```python
from build123d import *

# Parameters (mm, degrees)
F0_R     = 3.175
F1_DEPTH = 3.048


with BuildPart() as f1:
    # F0 (on Front) → F1 (new body)
    with BuildSketch(Plane.XZ):
        with BuildLine():
            Line((0.6794904459, -9.5007324841), (0, -9.525))
            ThreePointArc((0, -9.525), (0.3399618281, -9.5189311877), (0.6794904459, -9.5007324841))
        make_face()
        with BuildLine():
            Line((-15.7474569047, 61.4917106696), (-9.4773410414, -0.9516468803))
            ThreePointArc((-9.4773410414, -0.9516468803), (-7.0636414665, 6.3898821767), (0, 9.525))
            Line((0, 9.525), (0, 47.625))
            ThreePointArc((0, 47.625), (-10.4912828548, 51.5857812233), (-15.7474569047, 61.4917106696))
        make_face()
        with BuildLine():
            ThreePointArc((9.525, 0), (6.9712901065, -6.4905114784), (0.6794904459, -9.5007324841))
            Line((0.6794904459, -9.5007324841), (44.45, -7.9375))
            ThreePointArc((44.45, -7.9375), (38.8373399243, -5.6126600757), (36.5125, 0))
            Line((36.5125, 0), (9.525, 0))
        make_face()
        with BuildLine():
            Line((0, 104.775), (0, 79.375))
            ThreePointArc((0, 79.375), (10.4912828548, 75.4142187767), (15.7474569047, 65.5082893304))
            Line((15.7474569047, 65.5082893304), (9.525, 114.3))
            ThreePointArc((9.525, 114.3), (6.7351920908, 107.5648079092), (0, 104.775))
        make_face()
        with BuildLine():
            ThreePointArc((9.525, 114.3), (0, 123.825), (-9.525, 114.3))
            ThreePointArc((-9.525, 114.3), (-6.7351920908, 107.5648079092), (0, 104.775))
            ThreePointArc((0, 104.775), (6.7351920908, 107.5648079092), (9.525, 114.3))
        make_face()
        with BuildLine():
            ThreePointArc((3.175, 114.3), (2.2450640303, 112.0549359697), (0, 111.125))
            ThreePointArc((0, 111.125), (-2.2450640303, 116.5450640303), (3.175, 114.3))
        make_face(mode=Mode.SUBTRACT)
        with BuildLine():
            ThreePointArc((36.5125, 0), (38.8373399243, -5.6126600757), (44.45, -7.9375))
            ThreePointArc((44.45, -7.9375), (50.0626600757, -5.6126600757), (52.3875, 0))
            ThreePointArc((52.3875, 0), (50.0626600757, 5.6126600757), (44.45, 7.9375))
            ThreePointArc((44.45, 7.9375), (38.8373399243, 5.6126600757), (36.5125, 0))
        make_face()
        with BuildLine():
            ThreePointArc((47.625, 0), (44.45, -3.175), (41.275, 0))
            ThreePointArc((41.275, 0), (44.45, 3.175), (47.625, 0))
        make_face(mode=Mode.SUBTRACT)
        with BuildLine():
            Line((0, 60.325), (0, 47.625))
            ThreePointArc((0, 47.625), (10.4912828548, 51.5857812233), (15.7474569047, 61.4917106696))
            ThreePointArc((15.7474569047, 61.4917106696), (15.8430821396, 62.4938323604), (15.875, 63.5))
            ThreePointArc((15.875, 63.5), (15.8430821396, 64.5061676396), (15.7474569047, 65.5082893304))
            ThreePointArc((15.7474569047, 65.5082893304), (10.4912828548, 75.4142187767), (0, 79.375))
            Line((0, 79.375), (0, 66.675))
            ThreePointArc((0, 66.675), (2.2450640303, 65.7450640303), (3.175, 63.5))
            ThreePointArc((3.175, 63.5), (2.2450640303, 61.2549359697), (0, 60.325))
        make_face()
        with BuildLine():
            ThreePointArc((-15.7474569047, 65.5082893304), (-15.875, 63.5), (-15.7474569047, 61.4917106696))
            ThreePointArc((-15.7474569047, 61.4917106696), (-10.4912828548, 51.5857812233), (0, 47.625))
            Line((0, 47.625), (0, 60.325))
            ThreePointArc((0, 60.325), (-3.175, 63.5), (0, 66.675))
            Line((0, 66.675), (0, 79.375))
            ThreePointArc((0, 79.375), (-10.4912828548, 75.4142187767), (-15.7474569047, 65.5082893304))
        make_face()
        with BuildLine():
            Line((-9.525, 114.3), (-15.7474569047, 65.5082893304))
            ThreePointArc((-15.7474569047, 65.5082893304), (-10.4912828548, 75.4142187767), (0, 79.375))
            Line((0, 79.375), (0, 104.775))
            ThreePointArc((0, 104.775), (-6.7351920908, 107.5648079092), (-9.525, 114.3))
        make_face()
        with Locations((-6.35, 100.0252)):
            Circle(F0_R, mode=Mode.SUBTRACT)
        with BuildLine():
            Line((0, 47.625), (0, 9.525))
            ThreePointArc((0, 9.525), (6.7351920908, 6.7351920908), (9.525, 0))
            Line((9.525, 0), (36.5125, 0))
            ThreePointArc((36.5125, 0), (38.8373399243, 5.6126600757), (44.45, 7.9375))
            Line((44.45, 7.9375), (17.7825532299, 8.8935802069))
            ThreePointArc((17.7825532299, 8.8935802069), (12.0075791655, 11.6923910174), (10.1810740488, 17.8444269776))
            Line((10.1810740488, 17.8444269776), (15.7474569047, 61.4917106696))
            ThreePointArc((15.7474569047, 61.4917106696), (10.4912828548, 51.5857812233), (0, 47.625))
        make_face()
        with BuildLine():
            ThreePointArc((0, 9.525), (-7.0636414665, 6.3898821767), (-9.4773410414, -0.9516468803))
            ThreePointArc((-9.4773410414, -0.9516468803), (-6.3898821767, -7.0636414665), (0, -9.525))
            Line((0, -9.525), (0.6794904459, -9.5007324841))
            ThreePointArc((0.6794904459, -9.5007324841), (6.9712901065, -6.4905114784), (9.525, 0))
            Line((9.525, 0), (3.175, 0))
            ThreePointArc((3.175, 0), (-2.2450640303, -2.2450640303), (0, 3.175))
            Line((0, 3.175), (0, 9.525))
        make_face()
        with BuildLine():
            ThreePointArc((9.525, 0), (6.7351920908, 6.7351920908), (0, 9.525))
            Line((0, 9.525), (0, 3.175))
            ThreePointArc((0, 3.175), (2.2450640303, 2.2450640303), (3.175, 0))
            Line((3.175, 0), (9.525, 0))
        make_face()
    extrude(amount=F1_DEPTH)


solid = f1.part
```
Geometry: final body of the model. Coordinates: model frame, mm. A direction names the side the tool comes from. Coordinates: 2 decimals unless noted, no trailing zeros. Order: outer loops, then holes, each group sorted by start corner. A loop starts at its lowest first (then second) coordinate and runs counter-clockwise, first axis right, second up. Notation, with made-up numbers: (47, 5.25) - (91, 5.25) arc R20 cw to (91, 35.25) - close; hole circle Ø8 at (74, -3.75). An arc over 180 degrees is marked (long way). Write each question's results on one line, items separated by ' | '.
(1) Set-up query: faces 5 (the face through (0.209, -1.503, 123.823)), 6 (the face through (12.925, -1.503, 39.363)). Return all of +Z, -Z, +X, -X, +Y, -Y with unobstructed straight access to the full face (end or side cutting, diameter ignored); none if empty.
Values found:
face 5: +Z, +Y, -Y | face 6: +X, +Y, -Y
(2) Line query: line 1 (Z direction, x = -2, y = -2.8); line 2 (X direction, y = -0.85, z = 114.3) (3 decimals); line 3 (Z direction, x = -0.5, y = -0.75). Output: solid intervals per line, ascending. Write a range as [from, to].
Values found:
line 1: z = [-9.31, -2.47], [2.47, 61.03], [65.97, 111.83], [116.77, 123.61] | line 2: x = [-9.525, -3.175], [3.175, 9.525] | line 3: z = [-9.51, -3.14], [3.14, 60.36], [66.64, 111.16], [117.44, 123.81]
(3) Section query B-B, the plane z = 84.5. Return the cut outline in (x, y), plus the area to 3 significant figures.
Values found:
outline: (-13.33, -3.05) - (13.33, -3.05) - (13.33, 0) - (-13.33, 0) - close | area: 81.2 mm²
(4) Section query A-A, the plane y = -2.35. Count the separate pieces of the cut face and the enclosed holes in it, plus the area to 3 significant figures.
Values found:
separate pieces: 1 | enclosed holes: 5 | area: 3,730 mm²
(5) Mould query, pull axis X, two halves, no side actions, for faces 1 (the face through (-6.763, -1.503, 103.173)), 2 (the face through (-15.875, -1.503, 63.528)), 3 (the face through (41.52, -1.5, -1.22)), 4 (the face through (3, 0, 43)). Classes: +X half, -X half, draft (parallel to the pull), parting line (faces both ways), or undercut.
Values found:
face 1: undercut | face 2: -X half | face 3: undercut | face 4: draft
(6) Section query C-C, the plane x = 6.5. Return the cut outline in (y, z).
Values found:
outline: (-3.05, -9.29) - (0, -9.29) - (0, 121.26) - (-3.05, 121.26) - close
